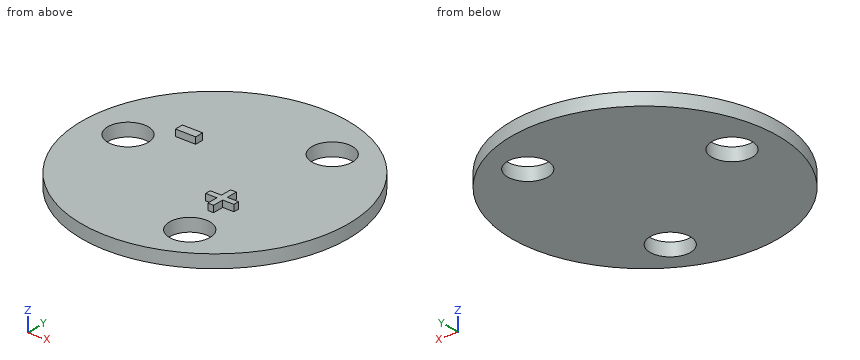
Autodesk Inventor part; units mm, degrees
ref_plane "YZ Plane" through (0, 0, 0) normal (1, 0, 0) x (0, 1, 0)
ref_plane "XZ Plane" through (0, 0, 0) normal (0, 1, 0) x (-1, 0, 0)
ref_plane "XY Plane" through (0, 0, 0) normal (0, 0, 1) x (1, 0, 0)
sketch "Skizze1" plane through (0, 0, 0) normal (0, 0, 1) x (1, 0, 0)
  circle A0 centre (0, 0) radius 20.4
  dimension "d0" = 40.8
extrude "Extrusion1" add sketch "Skizze1" against normal blind 2
sketch "Skizze2" plane through (0, 0, 0) normal (0, 0, 1) x (1, 0, 0)
  circle A0 centre (10.4908, -0.4387) radius 8.6464
  circle A1 centre (-5.6254, -8.866) radius 9
  circle A2 centre (-4.8655, 9.3047) radius 8.6464
  circle A3 centre (0, 0) radius 20.5
  circle A4 centre (-14.0161, 0.868) radius 3.1
  line L0 (-4.8655, 0.6582) -> (-4.8655, 0.1019) construction
  line L1 (-20.4642, 1.2118) -> (10.4908, -0.4387) construction
  circle A5 centre (6.2563, -12.5723) radius 3.1
  circle A6 centre (7.7598, 11.7043) radius 3.1
  point P0 (0, 0)
  point P1 (6.7426, -12.9951)
  point P2 (7.8827, 12.3368)
  dimension "d15" = 6.2
  dimension "d22" = 360
hole "Bohrung1" at (6.7426, -12.9951, 0) at (-14.0161, 0.868, 0) at (7.8827, 12.3368, 0) direction (0, 0, -1) diameter 6.2 end through all
sketch "Skizze3" plane through (0, 0, 0) normal (0, 0, 1) x (1, 0, 0)
  line L0 (2.9844, -3.6305) -> (8.6125, -3.6305) construction
  line L1 (8.6125, -3.6305) -> (8.6125, -10.4322) construction
  line L2 (8.6125, -10.4322) -> (2.9844, -10.4322) construction
  line L3 (2.9844, -10.4322) -> (2.9844, -3.6305) construction
  line L4 (-9.8763, 5.3535) -> (-5.1258, 5.3535) construction
  line L5 (-5.1258, 5.3535) -> (-5.1258, 3.2524) construction
  line L6 (-5.1258, 3.2524) -> (-9.8763, 3.2524) construction
  line L7 (-9.8763, 3.2524) -> (-9.8763, 5.3535) construction
  line L8 (7.9601, -6.2035) -> (6.2421, -6.2035)
  line L9 (6.2421, -6.2035) -> (6.2421, -7.9093)
  line L10 (6.2421, -7.9093) -> (5.3548, -7.9093)
  line L11 (5.3548, -7.9093) -> (5.3548, -6.2035)
  line L12 (5.3548, -6.2035) -> (3.6368, -6.2035)
  line L13 (3.6368, -6.2035) -> (3.6368, -5.3364)
  line L14 (3.6368, -5.3364) -> (5.3548, -5.3364)
  line L15 (5.3548, -5.3364) -> (5.3548, -3.6305)
  line L16 (5.3548, -3.6305) -> (6.2421, -3.6305)
  line L17 (6.2421, -3.6305) -> (6.2421, -5.3364)
  line L18 (6.2421, -5.3364) -> (7.9601, -5.3364)
  line L19 (7.9601, -5.3364) -> (7.9601, -6.2035)
  line L20 (-6.2458, 4.0488) -> (-9.3601, 4.0488)
  line L21 (-9.3601, 4.0488) -> (-9.3601, 5.3535)
  line L22 (-9.3601, 5.3535) -> (-6.2458, 5.3535)
  line L23 (-6.2458, 5.3535) -> (-6.2458, 4.0488)
  point P0 (0, 0)
extrude "Extrusion2" add sketch "Skizze3" along normal blind 1
properties part number "akkufach_deckel"
Geometry: final body of the model. Coordinates: model frame, mm. Give positions to 0.01 mm unless a question says otherwise; leave off trailing zeros. Write each loop counter-clockwise with the first axis right and the second up, starting at its lowest first coordinate (ties: lowest second). Pieces come first, ordered by that corner, then holes.
1. Section query B-B, the plane y = 0. Return loops of the section in (x, z), then the cut area to 3 significant figures.
2. Section query D-D, the plane z = -1. Return loops of the section in (x, y).
3. Section query C-C, the plane x = 0. Return loops of the section in (y, z), then the cut area to 3 significant figures.
4. Section query A-A, the plane x = -12. Return loops of the section in (y, z).
5. Pin query (flat end, axial travel): P1, Ø1.1, axis at x = 4, z = 0.5, coming from the +Y side; P2, Ø0.5, axis at y = 5, z = 0.5, coming from the -X side; P3, Ø10, axis at x = 4.5, y = -15, coming from the +Z side; P4, Ø20.5, axis at x = 5, y = 2, coming from the +Z side. Return the tip coordinate at first contact, or that it passes through.
6. Line query: probe 1 along Y at (x, z) = (9, -0.85); probe 2 along Y at (x, z) = (9.5, -1.35); probe 3 along Z at (x, y) = (-12, 16). Output: solid intervals per line, ascending.
Computed:
1. outline: (-20.4, -2) - (-16.99, -2) - (-16.99, 0) - (-20.4, 0) - close; (-11.04, -2) - (20.4, -2) - (20.4, 0) - (-11.04, 0) - close
1. area: 69.7 mm2
2. outline: circle Ø40.8 at (0, 0); hole circle Ø6.2 at (-14.02, 0.87); hole circle Ø6.2 at (6.74, -13); hole circle Ø6.2 at (7.88, 12.34)
3. outline: (-20.4, -2) - (20.4, -2) - (20.4, 0) - (-20.4, 0) - close
3. area: 81.6 mm2
4. outline: (-16.5, -2) - (-1.49, -2) - (-1.49, 0) - (-16.5, 0) - close; (3.22, -2) - (16.5, -2) - (16.5, 0) - (3.22, 0) - close
5. P1: stops at y = 20.05
5. P2: stops at x = -9.36
5. P3: stops at z = 0
5. P4: stops at z = 1
6. probe 1: y = -18.31 to -15.12, -10.87 to 9.45, 15.23 to 18.31
6. probe 2: y = -18.05 to -14.41, -11.58 to 9.69, 14.98 to 18.05
6. probe 3: z = -2 to 0
